Here's the drawing with two shaded views (mm, measured from the low corner). I have some questions. Round coordinates to 2 decimals unless told otherwise and drop trailing zeros. Order: outer loops, then holes, each group sorted by start corner. A loop starts at its lowest first (then second) coordinate and runs counter-clockwise, first axis right, second up. Notation, with made-up numbers: (32, 24.5) - (87, 24.5) arc R14 ccw to (87, 48.5) - close; hole circle Ø4 at (3.5, 28). An arc over 180 degrees is marked (long way). Return JSON: item names as keys, results as strings. Group by question number.
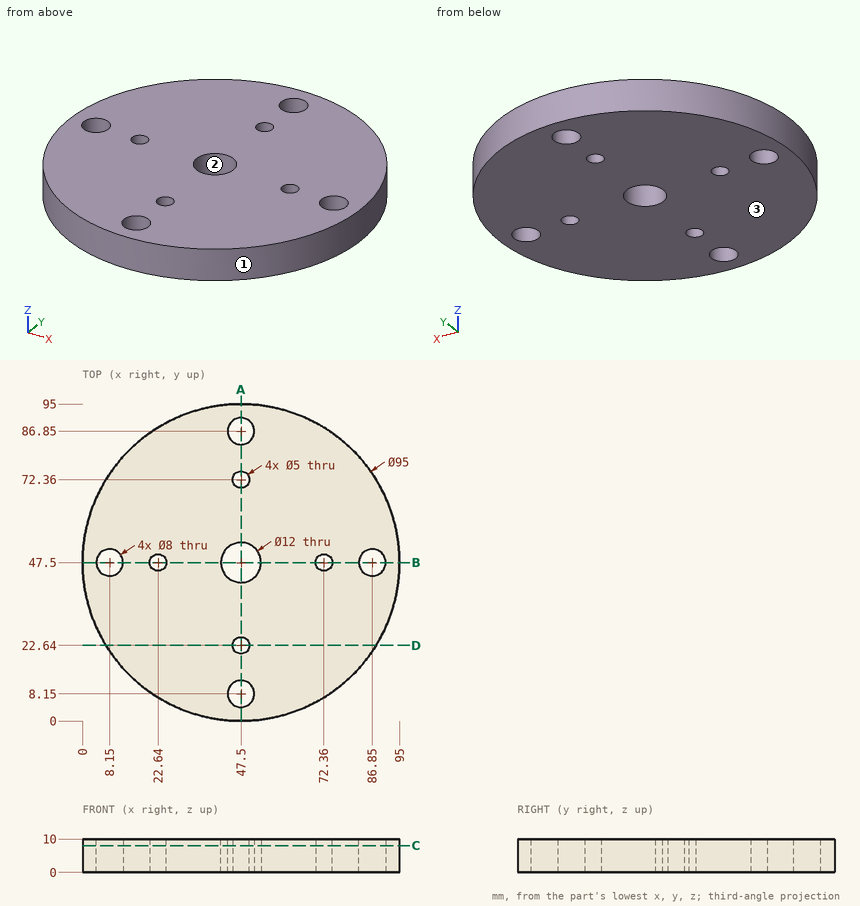
1) Will these pins go through, and if not, where does the flat tip stop? pin 1 (4 mm diameter, centred on x = 50, z = 9, fed in from -Y); pin 2 (1 mm diameter, centred on y = 82.5, z = 7, fed in from -X); pin 3 (1 mm diameter, centred on x = 11.5, z = 8, fed in from +Y).
2) If I drill on line 1 along Y through (x, z) = (47.5, 5); line 2 along Y through (x, z) = (47, 3.25); line 3 along X through (y, z) = (6, 2.25), over which ranges is the centre line in solid material (lowest first)? Write a range as from..to.
3) I want a section at A-A, the plane x = 47.5. List the corners of the cut face in (y, z) for me, plus the area to 3 significant figures.
4) I want a section at C-C, the plane z = 8. Give the number of separate pieces and of enclosed holes in the cut face, plus the area to 3 significant figures.
5) We'd pull the mould along X, two halves only. Please class the marked faces 1, 2 and 3: +X half, -X half, draft (parallel to the pull), parting line (faces both ways), or undercut.
6) I want a section at D-D, the plane y = 22.64. List the corners of the cut face in (x, z) for me, plus the area to 4 significant figures.
Outcome:
{
 "1": {"pin 1": "y = 0", "pin 2": "x = 14.85", "pin 3": "y = 79.06"},
 "2": {"line 1": "0..4.15, 12.15..20.14, 25.14..41.5, 53.5..69.86, 74.86..82.85, 90.85..95", "line 2": "0..4.18, 12.12..20.19, 25.09..41.52, 53.48..69.91, 74.81..82.88, 90.82..95", "line 3": "24.39..44.13, 50.87..70.61"},
 "3": {"outline": "(0, 0) - (4.15, 0) - (4.15, 10) - (0, 10) - close; (12.15, 0) - (20.14, 0) - (20.14, 10) - (12.15, 10) - close; (25.14, 0) - (41.5, 0) - (41.5, 10) - (25.14, 10) - close; (53.5, 0) - (69.86, 0) - (69.86, 10) - (53.5, 10) - close; (74.86, 0) - (82.85, 0) - (82.85, 10) - (74.86, 10) - close; (90.85, 0) - (95, 0) - (95, 10) - (90.85, 10) - close", "area": "570 mm^2"},
 "4": {"separate pieces": "1", "enclosed holes": "9", "area": "6,700 mm^2"},
 "5": {"face 1": "parting line", "face 2": "undercut", "face 3": "draft"},
 "6": {"outline": "(7.02, 0) - (45, 0) - (45, 10) - (7.02, 10) - close; (50, 0) - (87.98, 0) - (87.98, 10) - (50, 10) - close", "area": "759.5 mm^2"}
}
